Work out the finished part from the listing and answer in its coordinate system (mm). Round coordinates to 2 decimals unless told otherwise and drop trailing zeros. Write each loop counter-clockwise with the first axis right and the second up, starting at its lowest first coordinate (ties: lowest second). Pieces come first, ordered by that corner, then holes. Notation, with made-up numbers: (28.25, -2) -> (55.25, -2) arc R26 cw to (55.25, 24) -> close; hole circle Ø1 at (14, 68). An arc over 180 degrees is marked (long way). One line per item, written item: value.
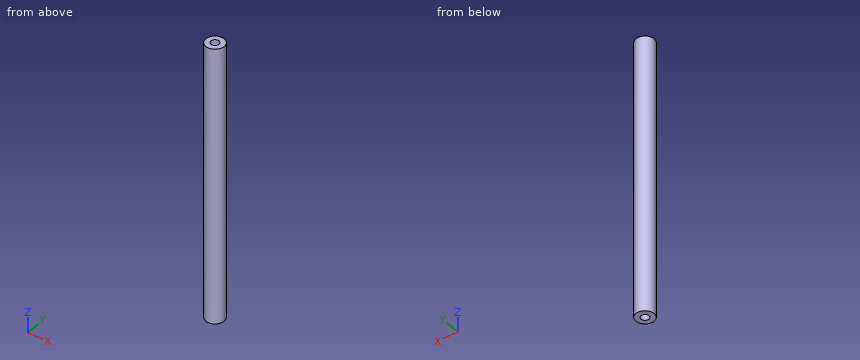
Autodesk Inventor part; units mm, degrees
ref_plane "YZ Plane" through (0, 0, 0) normal (1, 0, 0) x (0, 1, 0)
ref_plane "XZ Plane" through (0, 0, 0) normal (0, 1, 0) x (-1, 0, 0)
ref_plane "XY Plane" through (0, 0, 0) normal (0, 0, 1) x (1, 0, 0)
sketch "Sketch1" plane through (0, 0, 0) normal (0, 0, 1) x (1, 0, 0)
  circle A0 centre (0, 0) radius 2.5
  dimension "d0" = 5
extrude "Extrusion1" add sketch "Sketch1" along normal blind 75
sketch "Sketch2" plane through (0, 0, 75) normal (0, 0, 1) x (1, 0, 0)
  circle A0 centre (0, 0) radius 1.1
  dimension "d3" = 2.2
extrude "Extrusion2" cut sketch "Sketch2" against normal blind 20
sketch "Sketch3" plane through (0, 0, 0) normal (0, 0, -1) x (-1, 0, 0)
  circle A0 centre (0, 0) radius 1.1
extrude "Extrusion3" cut sketch "Sketch3" against normal blind 20
thread "Thread1"
thread "Thread2"
properties part number "AxisLinear"
(1) Find section D-D on z = 46. Give the vertices of the cut face in (x, y), plus the area to 3 significant figures.
Reported:
outline: circle Ø5 at (0, 0)
area: 19.6 mm2
(2) Find section A-A on x = 0. Give the vertices of the cut face in (y, z), plus the area to 3 significant figures.
Reported:
outline: (-2.5, 0) -> (-1.1, 0) -> (-1.1, 20) -> (1.1, 20) -> (1.1, 0) -> (2.5, 0) -> (2.5, 75) -> (1.1, 75) -> (1.1, 55) -> (-1.1, 55) -> (-1.1, 75) -> (-2.5, 75) -> close
area: 287 mm2
(3) Flat-ended cylindrical pins translate along their axes: pin 1 Ø1.8 at (x, y) = (0, 0) entering from -Z; pin 2 Ø1.5 at (x, z) = (1, 50.5) entering from -Y. Find the tip coordinate at first contact, or state that the pin passes through.
Reported:
pin 1: stops at z = 20
pin 2: stops at y = -2.49
(4) Consider probe 1 along Y at (x, z) = (0, 61.75); probe 2 along X at (y, z) = (0.2, 29.5); probe 3 along Z at (x, y) = (-0.1, 0.2). Determine where each line is inside the solid, lowest interval first.
Reported:
probe 1: y = -2.5 to -1.1, 1.1 to 2.5
probe 2: x = -2.49 to 2.49
probe 3: z = 20 to 55
(5) Find section C-C on z = 19. Give the vertices of the cut face in (x, y).
Reported:
outline: circle Ø5 at (0, 0); hole circle Ø2.2 at (0, 0)
